Read the model definition and answer for the solid it produces. Units are mm, in the model's axes. A direction names the side the tool comes from. Give positions to 0.01 mm unless a question says otherwise; leave off trailing zeros. Write each loop counter-clockwise with the first axis right and the second up, starting at its lowest first coordinate (ties: lowest second). Pieces come first, ordered by that corner, then holes. Notation, with made-up numbers: (57, 84) -> (99, 84) arc R7 ccw to (99, 92) -> close; hole circle Ø2 at (65, 6). An arc over 180 degrees is marked (long way). Use a Markdown table: item, result.
Autodesk Inventor part; units mm, degrees
ref_plane "YZ Plane" through (0, 0, 0) normal (1, 0, 0) x (0, 1, 0)
ref_plane "XZ Plane" through (0, 0, 0) normal (0, 1, 0) x (-1, 0, 0)
ref_plane "XY Plane" through (0, 0, 0) normal (0, 0, 1) x (1, 0, 0)
sketch "Sketch1" plane through (0, 0, 0) normal (0, 0, 1) x (1, 0, 0)
  circle A0 centre (0, 0) radius 11
  line L0 (9.8023, 37.5977) -> (3, 35.24)
  line L1 (3, 35.24) -> (3, 11.34)
  line L2 (3, 11.34) -> (9, 11.34)
  line L3 (9, 11.34) -> (9, 30.1331)
  line L4 (9, 30.1331) -> (7.9327, 24.5668)
  line L5 (7.9327, 24.5668) -> (7.3445, 24.6796)
  line L6 (7.3445, 24.6796) -> (9.8023, 37.5977)
  circle A1 centre (0, 0) radius 12.5167
  line L7 (-21, 24.5198) -> (-21, -3.96)
  line L8 (-19, -3.96) -> (-21, -3.96)
  line L9 (-19, 24.5198) -> (-19, -3.96)
  line L10 (-21, 24.5198) -> (-19, 24.5198)
  line L11 (-21, 28.5732) -> (-21, 24.5198)
  line L12 (-21, 24.5198) -> (-19, 24.5198)
  line L13 (-19, 28.5732) -> (-19, 24.5198)
  line L14 (-21, 28.5732) -> (-19, 28.5732)
  line L15 (1.6453, 33.2633) -> (-11.4547, 33.2633)
  line L16 (-19, 0.49) -> (-19, -3.96)
  line L17 (-14, 0.49) -> (-19, 0.49)
  line L18 (-14, -0.96) -> (-14, 0.49)
  arc A2 (-14, -0.96) -> (-11, -3.96) centre (-11, -0.96) ccw
  line L19 (-11, -3.96) -> (-19, -3.96)
  line L20 (3, 35.24) -> (-21, 35.24)
  line L21 (-11.4547, 35.24) -> (-22.0722, 28.5732)
  line L22 (-22.0722, 28.5732) -> (-23.4016, 30.6904)
  line L23 (-23.4016, 30.6904) -> (-12.7841, 37.3572)
  line L24 (-23.4016, 30.6904) -> (-25.0875, 29.6318)
  line L25 (-25.0875, 29.6318) -> (-25.0875, -6.2453)
  line L26 (-25.0875, -6.2453) -> (-5.3307, -11.3248)
  point P0 (0, 0)
  point P1 (3, 12.1518)
  point P2 (-16.156, 35.24)
  dimension "d0" = 2.5
extrude "Extrusion1" add sketch "Sketch1" against normal blind 3 contours L1 A1 A2 L18 L17 L9 L13 L14 L11 L7 L8 L19 L26 L25 L24 L22 L21 L20 | L21 L22 L23 L20 | A1 L19 L9 L17 L18 A2 | L8 L7 L10 L9 | L11 L14 L13 L10
ref_plane "Work Plane1" through (0, 0, -50) normal (0, 0, -1) x (1, 0, 0)
sketch "Sketch2" plane through (0, 0, -50) normal (0, 0, -1) x (1, 0, 0)
  line L0 (3, -35.24) -> (3, -12.1518)
  arc A0 (-5.3307, 11.3248) -> (3, -12.1518) centre (0, 0) ccw
  line L1 (-5.3307, 11.3248) -> (-25.0875, 6.2453)
  line L2 (-25.0875, 6.2453) -> (-25.0875, -29.6318)
  line L3 (-25.0875, -29.6318) -> (-16.156, -35.24)
  line L4 (-16.156, -35.24) -> (3, -35.24)
  point P0 (0, 0)
extrude "Extrusion2" add sketch "Sketch2" against normal blind 3
sketch "Sketch3" plane through (0, 0, -47) normal (0, 0, 1) x (1, 0, 0)
  line L0 (-25.0875, 29.6318) -> (-25.0875, -6.2453)
  line L1 (-25.0875, -6.2453) -> (-5.3307, -11.3248)
  arc A0 (3, 12.1518) -> (-5.3307, -11.3248) centre (0, 0) ccw
  line L2 (3, 12.1518) -> (3, 35.24)
  line L3 (3, 35.24) -> (-16.156, 35.24)
  line L4 (-16.156, 35.24) -> (-25.0875, 29.6318)
  line L5 (-25.0875, 29.6318) -> (-25.0875, -6.2453)
  line L6 (-25.0875, -6.2453) -> (-22.5875, -6.2453)
  line L7 (-22.5875, -6.2453) -> (-22.5875, 29.6318)
  line L8 (-22.5875, 29.6318) -> (-25.0875, 29.6318)
  line L9 (-25.0875, 29.6318) -> (-25.0875, -6.2453)
  line L10 (-16.156, 35.24) -> (-25.0875, 29.6318)
  line L11 (-20.6218, 32.4359) -> (-19.2923, 30.3187)
  line L12 (-19.2923, 30.3187) -> (-10.0223, 36.1394)
  line L13 (-10.0223, 36.1394) -> (-28.1615, 24.7497)
  line L14 (3, 12.1518) -> (3, 35.24)
  line L15 (3, 35.24) -> (-20.6218, 35.24)
  line L16 (-20.6218, 35.24) -> (-20.6218, 32.74)
  line L17 (-20.6218, 32.74) -> (3, 32.74)
  line L18 (3, 32.74) -> (3, 35.24)
  line L19 (-25.0875, -6.2453) -> (-5.3307, -11.3248)
  line L20 (-15.2091, -8.7851) -> (-14.5866, -6.3638)
  line L21 (-14.5866, -6.3638) -> (-34.8376, -1.1573)
  line L22 (-14.5866, -6.3638) -> (7.6026, -12.0686)
  point P0 (0, 0)
  point P1 (-9.9857, -7.5467)
  point P2 (-22.5875, -4.3067)
  point P3 (-22.5875, 28.2496)
  point P4 (-15.4362, 32.74)
  point P5 (3, 32.74)
  dimension "d5" = 2.5
  dimension "d6" = 2.5
  dimension "d7" = 2.5
  dimension "d8" = 2.5
extrude "Extrusion3" add sketch "Sketch3" along normal up to surface (44 mm away) contours L8 L7 L13 L0 | L4 L11 L13 L7 L8 | L13 L7 L21 L0 | L4 L17 L12 L11 | L21 L7 L6 L0 | L4 L3 L12 L17 | L6 L7 L21 L20 L1 | L12 L3 L2 L17 | L20 L22 A0 L1
sketch "Sketch4" plane through (-16.156, 35.24, 0) normal (0, 1, 0) x (1, 0, 0)
  line L0 (19.156, 0) -> (0, 0)
  line L1 (19.156, 0) -> (19.156, 50)
  line L2 (0, 50) -> (19.156, 50)
  line L3 (0, 0) -> (0, 50)
  line L4 (18.4023, 21.528) -> (18.4023, 31.928)
  line L5 (5.3023, 21.528) -> (18.4023, 21.528)
  line L6 (5.3023, 31.928) -> (5.3023, 21.528)
  line L7 (18.4023, 31.928) -> (5.3023, 31.928)
  line L8 (5.039, 38.3353) -> (18.139, 38.3353)
  line L9 (18.139, 38.3353) -> (18.139, 47.6905)
  line L10 (5.039, 38.3353) -> (18.139, 38.3353)
  line L11 (18.139, 38.3353) -> (18.139, 47.6905)
  line L12 (5.039, 38.3353) -> (18.139, 38.3353)
  line L13 (5.039, 47.6905) -> (5.039, 38.3353)
  line L14 (18.139, 47.6905) -> (5.039, 47.6905)
  line L15 (17.8013, 2.855) -> (17.8013, 11.7262)
  line L16 (4.7013, 2.855) -> (17.8013, 2.855)
  line L17 (4.7013, 11.7262) -> (4.7013, 2.855)
  line L18 (17.8013, 11.7262) -> (4.7013, 11.7262)
  line L19 (18.4023, 21.528) -> (18.4023, 31.928)
  line L20 (5.3023, 21.528) -> (18.4023, 21.528)
  line L21 (5.3023, 31.928) -> (5.3023, 21.528)
  line L22 (18.4023, 31.928) -> (5.3023, 31.928)
  line L23 (5.039, 39.2089) -> (18.139, 39.2089)
  line L24 (18.139, 39.2089) -> (18.139, 48.5642)
  line L25 (17.8013, 1.8112) -> (17.8013, 10.6824)
  line L26 (17.8013, 11.7262) -> (17.8013, 10.6824)
  line L27 (17.8013, 11.7262) -> (4.7013, 11.7262)
  line L28 (17.8013, 1.8112) -> (17.8013, 10.6824)
  line L29 (17.8013, 2.855) -> (17.8013, 1.8112)
  point P0 (16.156, 0)
extrude "Extrusion4" cut sketch "Sketch4" against normal blind 10 contours L5 L6 L7 L4 | L13 L23 L9 L8 | L13 L14 L9 L23 | L16 L17 L18 L15
sketch "Sketch5" plane through (0, 0, -50) normal (0, 0, -1) x (-1, 0, 0)
  line L0 (25.0875, -6.2453) -> (25.0875, 29.6318)
  line L1 (25.0875, 29.6318) -> (16.156, 35.24)
  line L2 (16.156, 35.24) -> (-3, 35.24)
  line L3 (-3, 35.24) -> (-3, 12.1518)
  arc A0 (5.3307, -11.3248) -> (-3, 12.1518) centre (0, 0) ccw
  line L4 (5.3307, -11.3248) -> (25.0875, -6.2453)
  arc A1 (9.9857, -7.5467) -> (-3, 12.1518) centre (0, 0) ccw
  line L5 (12.5167, 0) -> (12.5167, -6.898)
  line L6 (25.0875, -6.2453) -> (15.0147, -8.835)
  line L7 (5.3307, -11.3248) -> (25.0875, -6.2453)
  arc A2 (12.5167, -6.898) -> (15.0147, -8.835) centre (14.5167, -6.898) ccw
  point P0 (0, 0)
  point P1 (12.5167, -9.4773)
  point P2 (15.0147, -8.835)
  point P3 (12.5167, 0)
  dimension "d13" = 2
extrude "Extrusion5" cut sketch "Sketch5" against normal through all contours L4 A0 L5 A2
properties part number "obudowa"
Item 1: A cutting plane is placed at B-B (x = -21.5). Give the vertices of the cut face in (y, z).
Return value:
| item | result |
|---|---|
| outline | (-7.17, -50) -> (31.88, -50) -> (31.88, 0) -> (-7.17, 0) -> close; hole (-4.59, -47) -> (28.93, -47) -> (28.93, -3) -> (-4.59, -3) -> close |
Item 2: A cutting plane is placed at D-D (x = 0.5). Count the separate pieces of the cut face and the enclosed holes in it, then the cut area to 3 significant figures.
Return value:
| item | result |
|---|---|
| separate pieces | 4 |
| enclosed holes | 0 |
| area | 169 mm^2 |
Item 3: Straight lines are drawn through the part: line 1 along Z through (x, y) = (-17.5, 25.5); line 2 along Z through (x, y) = (1, 26) (1 decimal); line 3 along Y through (x, z) = (-11.5, -14). For each, find the intervals that lie inside material, in ascending order. Write a range as [from, to].
Return value:
| item | result |
|---|---|
| line 1 | [-50, -47], [-3, 0] |
| line 2 | [-50, -47.7], [-2.9, 0] |
| line 3 | [32.74, 35.24] |
Item 4: A cutting plane is placed at A-A (y = -3.5). Give the vertices of the cut face in (x, z), then the cut area to 3 significant figures.
Return value:
| item | result |
|---|---|
| outline | (-25.09, -50) -> (-12.52, -50) -> (-12.52, -47) -> (-22.59, -47) -> (-22.59, -3) -> (-12.52, -3) -> (-12.52, 0) -> (-25.09, 0) -> close |
| area | 185 mm^2 |
Item 5: A tool of negligible diameter and unlimited length cuts with its end or side. For faces 4 (the face through (-13, 13, -3)), 5 (the face through (-11.117, 33, -44)), 6 (the face through (-19.98, -7.56, -25.35)), 7 (the face through (-9, 35.24, -20)), 8 (the face through (-4, 34, -21.528)), from which of +Z, -Z, +X, -X, +Y, -Y can it reach the whole face along a straight path? Write none if from no direction.
Return value:
| item | result |
|---|---|
| face 4 | +X |
| face 5 | +Y |
| face 6 | +Z, -Z, -X, -Y |
| face 7 | +Z, -Z, +X, -X, +Y |
| face 8 | +Y, -Y |
Item 6: Each of these flat-tipped pins is pushed along its axis until it touches: P1, Ø0.8, axis at x = -4.5, z = -47, coming from the +Y side; P2, Ø10, axis at x = -1.5, z = -20, coming from the -Y side; P3, Ø1.5, axis at x = -20, z = -18, coming from the -Y side. Where does it stop, or does it pass through?
Return value:
| item | result |
|---|---|
| P1 | y = 25.24 |
| P2 | y = 32.74 |
| P3 | y = -7.75 |
Item 7: For a pull along Z with two mould halves and no side action, classify faces 1 (the face through (-5, 34, -38.335)), 2 (the face through (-7.842, 9.756, -48.521)), 3 (the face through (-11, 18, -50)) as +Z half, -Z half, draft (parallel to the pull), parting line (faces both ways), or undercut.
Return value:
| item | result |
|---|---|
| face 1 | undercut |
| face 2 | draft |
| face 3 | -Z half |
